from build123d import *

# Parameters (mm, degrees)
F1_DEPTH = 30
F0_W     = 15
F0_H     = 20
F2_DEPTH = 15
F5_DEPTH = 25.001


with BuildPart() as f1:
    # F0 (on Top) → F1 (new body)
    with BuildSketch(Plane.XY):
        Polygon((-39.3988706533, 18.9813024559), (-54.3988706533, 18.9813024559), (-54.3988706533, -16.0186975441), (5.6011293467, -16.0186975441), (5.6011293467, -6.0186975441), (65.6011293467, -6.0186975441), (65.6011293467, 8.9813024559), (50.6011293467, 8.9813024559), (-39.3988706533, 8.9813024559), align=None)
    extrude(amount=F1_DEPTH)

    # F0 (on Top) → F2 (join)
    with BuildSketch(Plane.XY):
        Polygon((-39.3988706533, 18.9813024559), (-54.3988706533, 18.9813024559), (-54.3988706533, -16.0186975441), (5.6011293467, -16.0186975441), (5.6011293467, -6.0186975441), (65.6011293467, -6.0186975441), (65.6011293467, 8.9813024559), (50.6011293467, 8.9813024559), (-39.3988706533, 8.9813024559), align=None)
        with Locations((58.1011293467, 18.9813024559)):
            Rectangle(F0_W, F0_H)
    extrude(amount=F2_DEPTH)

    # F3: F1 across face


with BuildPart() as f1_1:
    add(f1.part)
    add(f1.part.mirror(Plane(origin=(-4.5459294768, -0.7245798971, 30), x_dir=(1, 0, 0), z_dir=(0, 0, 1))))

    # F4 (on face) → F5 (cut, through all)
    with BuildSketch(Plane(origin=(0, 8.9813024559, 0), x_dir=(-1, 0, 0), z_dir=(0, 1, 0))):
        with BuildLine():
            Line((-30.6011293467, 20), (-30.6011293467, 30))
            Line((-30.6011293467, 30), (-40.6011293467, 30))
            ThreePointArc((-40.6011293467, 30), (-37.6721971586, 22.9289321881), (-30.6011293467, 20))
        make_face()
        with BuildLine():
            Line((-20.6011293467, 30), (-30.6011293467, 30))
            Line((-30.6011293467, 30), (-30.6011293467, 20))
            ThreePointArc((-30.6011293467, 20), (-23.5300615349, 22.9289321881), (-20.6011293467, 30))
        make_face()
        with BuildLine():
            ThreePointArc((-20.6011293467, 30), (-23.5300615349, 37.0710678119), (-30.6011293467, 40))
            Line((-30.6011293467, 40), (-30.6011293467, 30))
            Line((-30.6011293467, 30), (-20.6011293467, 30))
        make_face()
        with BuildLine():
            Line((-30.6011293467, 30), (-30.6011293467, 40))
            ThreePointArc((-30.6011293467, 40), (-37.6721971586, 37.0710678119), (-40.6011293467, 30))
            Line((-40.6011293467, 30), (-30.6011293467, 30))
        make_face()
        with BuildLine():
            Line((24.3988706533, 30), (14.3988706533, 30))
            Line((14.3988706533, 30), (14.3988706533, 20))
            ThreePointArc((14.3988706533, 20), (21.4699384651, 22.9289321881), (24.3988706533, 30))
        make_face()
        with BuildLine():
            Line((14.3988706533, 30), (4.3988706533, 30))
            ThreePointArc((4.3988706533, 30), (7.3278028414, 22.9289321881), (14.3988706533, 20))
            Line((14.3988706533, 20), (14.3988706533, 30))
        make_face()
        with BuildLine():
            Line((14.3988706533, 30), (14.3988706533, 40))
            ThreePointArc((14.3988706533, 40), (7.3278028414, 37.0710678119), (4.3988706533, 30))
            Line((4.3988706533, 30), (14.3988706533, 30))
        make_face()
        with BuildLine():
            ThreePointArc((24.3988706533, 30), (21.4699384651, 37.0710678119), (14.3988706533, 40))
            Line((14.3988706533, 40), (14.3988706533, 30))
            Line((14.3988706533, 30), (24.3988706533, 30))
        make_face()
    extrude(amount=-F5_DEPTH, mode=Mode.SUBTRACT)


solid = f1_1.part
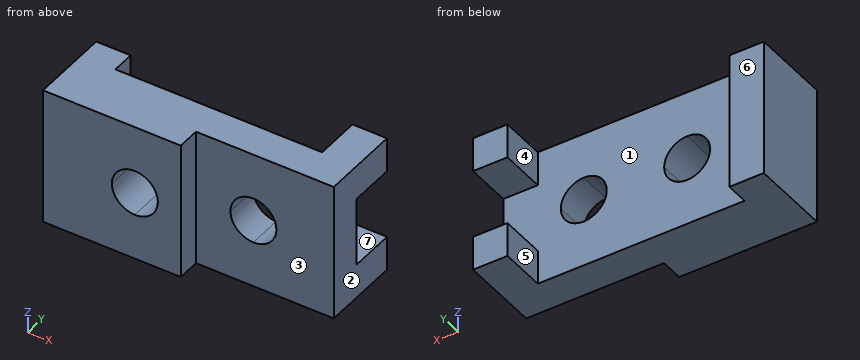
Here's how the part is built. I have some questions about the finished solid (model axes, mm). Face numbers are marked on the shaded views. A direction names the side the tool comes from. Round coordinates to 2 decimals unless told otherwise and drop trailing zeros. Order: outer loops, then holes, each group sorted by start corner. A loop starts at its lowest first (then second) coordinate and runs counter-clockwise, first axis right, second up. Notation, with made-up numbers: (-4, 59) -> (53, 59) arc R11 ccw to (53, 64) -> close; hole circle Ø1 at (-20, -21). An arc over 180 degrees is marked (long way). Return JSON: item names as keys, results as strings.
Q1. If we mould it in two halves opening along X, with no side actions, what happens to the marked faces 1, 2, 3 and 4? For each: released by +X, released by -X, zero draft, split by the parting line, or undercut.
Filled sheet:
{"face 1": "undercut", "face 2": "released by +X", "face 3": "zero draft", "face 4": "undercut"}
Q2. For pin 1 Ø4.5 at (x, z) = (-49, 21.5) entering from +Y; pin 2 Ø1.5 at (x, z) = (22.5, 22.5) entering from +Y; pin 3 Ø5 at (y, z) = (-9, 22.5) entering from +X, each with a flat end and sliding along its axis, tell me the tip position at first contact or that it passes through.
Filled sheet:
{"pin 1": "stops at y = 18.98", "pin 2": "stops at y = 8.98", "pin 3": "stops at x = 5.6"}
Q3. If we section it at B-B on y = 15: List the corners of the cut face in (x, z) for me.
Filled sheet:
{"outline": "(-54.4, 0) -> (-39.4, 0) -> (-39.4, 60) -> (-54.4, 60) -> close; (50.6, 0) -> (65.6, 0) -> (65.6, 15) -> (50.6, 15) -> close; (50.6, 45) -> (65.6, 45) -> (65.6, 60) -> (50.6, 60) -> close"}
Q4. If we section it at A-A on y = -0.5: List the corners of the cut face in (x, z) for me.
Filled sheet:
{"outline": "(-54.4, 0) -> (65.6, 0) -> (65.6, 60) -> (-54.4, 60) -> close; hole circle Ø20 at (-14.4, 30); hole circle Ø20 at (30.6, 30)"}
Q5. I need wall thicknesses on line 1 along X through (y, z) = (15, 5); line 2 along X through (y, z) = (-4.5, 22.5); line 3 along Z through (x, y) = (53, 20). Which ranges of each line are inside material? Lowest first, please. Write a range as from..to.
Filled sheet:
{"line 1": "x = -54.4..-39.4, 50.6..65.6", "line 2": "x = -54.4..-21.01, -7.78..23.99, 37.22..65.6", "line 3": "z = 0..15, 45..60"}
Q6. Which directions (+Z, -Z, +X, -X, +Y, -Y) give clear straight access to the entire face, cutting with the end or side of a thin tool? Please do the marked faces 5, 6 and 7.
Filled sheet:
{"face 5": "+Z, -Z, +Y", "face 6": "+Z, -Z, -X, +Y", "face 7": "+X, +Y"}
Q7. If we section it at D-D on x = 54.5: List the corners of the cut face in (y, z) for me.
Filled sheet:
{"outline": "(-6.02, 0) -> (28.98, 0) -> (28.98, 15) -> (8.98, 15) -> (8.98, 45) -> (28.98, 45) -> (28.98, 60) -> (-6.02, 60) -> close"}
Q8. If we section it at C-C on z = 51.5: List the corners of the cut face in (x, y) for me.
Filled sheet:
{"outline": "(-54.4, -16.02) -> (5.6, -16.02) -> (5.6, -6.02) -> (65.6, -6.02) -> (65.6, 28.98) -> (50.6, 28.98) -> (50.6, 8.98) -> (-39.4, 8.98) -> (-39.4, 18.98) -> (-54.4, 18.98) -> close"}
